Read the model definition and answer for the solid it produces. Units are mm, in the model's axes. Face numbers are marked on the shaded views. Coordinates: 2 decimals unless noted, no trailing zeros. Loops run counter-clockwise (first coordinate to the right, second up) from the corner with the lowest first, then second, coordinate; pieces in that order, holes last. Notation, with made-up numbers: (76, 62.25) -> (125, 62.25) arc R32 cw to (125, 100.25) -> close; hole circle Ø8 at (84.5, -12). An arc over 180 degrees is marked (long way). Answer in a Markdown table with one row per item.
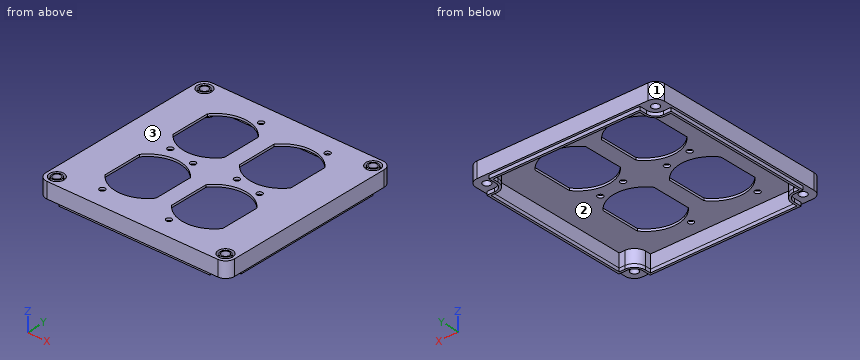
```python
from build123d import *

# Parameters (mm, degrees)
SKETCH1_W                 = 85
SKETCH1_H                 = 85
BOSS_EXTRUDE1_DEPTH       = 7
CUT_EXTRUDE4_DEPTH        = 6
FILLET4_R                 = 4
CUT_EXTRUDE1_DEPTH        = 61.510329697
SKETCH3_R                 = 1.25
CUT_EXTRUDE6_DEPTH        = 61.510329697
LPATTERN1_COUNT           = 2
LPATTERN1_PITCH           = 35
LPATTERN1_COUNT_DIR2      = 2
LPATTERN1_PITCH_DIR2      = 30
BOSS_EXTRUDE6_DEPTH       = 7
SKETCH15_R                = 1.75
CUT_EXTRUDE7_DEPTH        = 61.510329697
SKETCH30_R                = 3.25
CUT_EXTRUDE8_DEPTH        = 2
SKETCH31_R                = 2.25
SKETCH31_R_2              = 1.75
EXTRUDE_THIN2_DEPTH       = 2
MIRROR4_COPY_1_DEPTH      = 7
MIRROR4_COPY_2_SKETCH_R   = 1.75
MIRROR4_COPY_2_DEPTH      = 61.510329697
MIRROR4_COPY_3_SKETCH_R   = 3.25
MIRROR4_COPY_3_DEPTH      = 2
MIRROR4_COPY_4_SKETCH_R   = 2.25
MIRROR4_COPY_4_SKETCH_R_2 = 1.75
MIRROR4_COPY_4_DEPTH      = 2
MOVE_FACE1_BY             = 0.5
MOVE_FACE1_2_BY           = 0.5
MOVE_FACE1_3_BY           = 0.5
MOVE_FACE1_4_BY           = 0.5
MOVE_FACE1_5_BY           = 0.5
MOVE_FACE1_6_BY           = 0.5
MOVE_FACE1_7_BY           = 0.5
MOVE_FACE1_8_BY           = 0.5
MOVE_FACE1_9_BY           = 0.5
MOVE_FACE1_10_BY          = 0.5
MOVE_FACE1_11_BY          = 0.5
MOVE_FACE1_12_BY          = 0.5
EXTRUDE_THIN1_DEPTH       = 1.5


with BuildPart() as part:
    # Sketch1 → Boss-Extrude1 (new body)
    with BuildSketch(Plane.XY):
        Rectangle(SKETCH1_W, SKETCH1_H)
    extrude(amount=BOSS_EXTRUDE1_DEPTH)

    # Sketch8 → Cut-Extrude4 (cut)
    with BuildSketch(Plane(origin=(0, 0, 0), x_dir=(-1, 0, 0), z_dir=(0, 0, -1))):
        with BuildLine():
            Line((40.5, -37.5), (40.5, 37.5))
            ThreePointArc((40.5, 37.5), (39.621320344, 39.621320344), (37.5, 40.5))
            Line((37.5, 40.5), (-37.5, 40.5))
            ThreePointArc((-37.5, 40.5), (-39.621320344, 39.621320344), (-40.5, 37.5))
            Line((-40.5, 37.5), (-40.5, -37.5))
            ThreePointArc((-40.5, -37.5), (-39.621320344, -39.621320344), (-37.5, -40.5))
            Line((-37.5, -40.5), (37.5, -40.5))
            ThreePointArc((37.5, -40.5), (39.621320344, -39.621320344), (40.5, -37.5))
        make_face()
    extrude(amount=-CUT_EXTRUDE4_DEPTH, mode=Mode.SUBTRACT)

    # Fillet4
    fillet4_edges = [part.edges().sort_by_distance(p)[0] for p in [
        (42.5, -42.5, 3.5),
        (-42.5, -42.5, 3.5),
        (-42.5, 42.5, 3.5),
        (42.5, 42.5, 3.5),
    ]]
    fillet(fillet4_edges, radius=FILLET4_R)

    # Sketch2 → Cut-Extrude1 (cut, through all)
    with BuildSketch(Plane.XY.offset(7)):
        with BuildLine():
            Line((-26.5, 8.668239134), (-26.5, 26.331760866))
            ThreePointArc((-26.5, 26.331760866), (-15, 32), (-3.5, 26.331760866))
            Line((-3.5, 26.331760866), (-3.5, 8.668239134))
            ThreePointArc((-3.5, 8.668239134), (-15, 3), (-26.5, 8.668239134))
        make_face()
    cut_extrude1 = extrude(amount=-CUT_EXTRUDE1_DEPTH, mode=Mode.SUBTRACT)

    # Sketch3 → Cut-Extrude6 (cut, through all)
    with BuildSketch(Plane.XY.offset(7)):
        with Locations((-9, 34)):
            Circle(SKETCH3_R)
        with Locations((-21, 1)):
            Circle(SKETCH3_R)
    cut_extrude6 = extrude(amount=-CUT_EXTRUDE6_DEPTH, mode=Mode.SUBTRACT)

    # LPattern1: Cut-Extrude1, Cut-Extrude6 2 × 2
    with Locations(*[(j * LPATTERN1_PITCH_DIR2, -i * LPATTERN1_PITCH, 0) for i in range(LPATTERN1_COUNT) for j in range(LPATTERN1_COUNT_DIR2) if (i, j) != (0, 0)]):
        add(cut_extrude1, mode=Mode.SUBTRACT)
        add(cut_extrude6, mode=Mode.SUBTRACT)

    # Sketch14 → Boss-Extrude6 (add)
    with BuildSketch(Plane.XY.offset(7)):
        with BuildLine():
            Line((-38, 33.5), (-42.5, 33.5))
            Line((-42.5, 33.5), (-42.5, 38))
            ThreePointArc((-42.5, 38), (-41.181980515, 41.181980515), (-38, 42.5))
            Line((-38, 42.5), (-33.5, 42.5))
            Line((-33.5, 42.5), (-33.5, 38))
            ThreePointArc((-33.5, 38), (-34.818019485, 34.818019485), (-38, 33.5))
        make_face()
    boss_extrude6 = extrude(amount=-BOSS_EXTRUDE6_DEPTH)

    # Sketch15 → Cut-Extrude7 (cut, through all)
    with BuildSketch(Plane(origin=(0, 0, 0), x_dir=(-1, 0, 0), z_dir=(0, 0, -1))):
        with Locations((38, 38)):
            Circle(SKETCH15_R)
    cut_extrude7 = extrude(amount=-CUT_EXTRUDE7_DEPTH, mode=Mode.SUBTRACT)

    # Sketch30 → Cut-Extrude8 (cut)
    with BuildSketch(Plane.XY.offset(7)):
        with Locations((-38, 38)):
            Circle(SKETCH30_R)
    cut_extrude8 = extrude(amount=-CUT_EXTRUDE8_DEPTH, mode=Mode.SUBTRACT)

    # Sketch31 → Extrude-Thin2 (add)
    with BuildSketch(Plane.XY.offset(5)):
        with Locations((-38, 38)):
            Circle(SKETCH31_R)
        with Locations((-38, 38)):
            Circle(SKETCH31_R_2, mode=Mode.SUBTRACT)
    extrude_thin2 = extrude(amount=EXTRUDE_THIN2_DEPTH)

    # Mirror3: Boss-Extrude6, Cut-Extrude7, Cut-Extrude8, Extrude-Thin2 across plane
    add(boss_extrude6.mirror(Plane(origin=(0, 0, 0), x_dir=(0, 0, 1), z_dir=(1, 0, 0))))
    add(cut_extrude7.mirror(Plane(origin=(0, 0, 0), x_dir=(0, 0, 1), z_dir=(1, 0, 0))), mode=Mode.SUBTRACT)
    add(cut_extrude8.mirror(Plane(origin=(0, 0, 0), x_dir=(0, 0, 1), z_dir=(1, 0, 0))), mode=Mode.SUBTRACT)
    add(extrude_thin2.mirror(Plane(origin=(0, 0, 0), x_dir=(0, 0, 1), z_dir=(1, 0, 0))))

    # Mirror4: Boss-Extrude6, Cut-Extrude7, Cut-Extrude8, Extrude-Thin2 across plane
    add(boss_extrude6.mirror(Plane.ZX))
    add(cut_extrude7.mirror(Plane.ZX), mode=Mode.SUBTRACT)
    add(cut_extrude8.mirror(Plane.ZX), mode=Mode.SUBTRACT)
    add(extrude_thin2.mirror(Plane.ZX))

    # Mirror4 copy 1 sketch → Mirror4 copy 1 (add)
    with BuildSketch(Plane(origin=(0, 0, 7), x_dir=(-1, 0, 0), z_dir=(0, 0, 1))):
        with BuildLine():
            Line((-38, 33.5), (-42.5, 33.5))
            Line((-42.5, 33.5), (-42.5, 38))
            ThreePointArc((-42.5, 38), (-41.181980515, 41.181980515), (-38, 42.5))
            Line((-38, 42.5), (-33.5, 42.5))
            Line((-33.5, 42.5), (-33.5, 38))
            ThreePointArc((-33.5, 38), (-34.818019485, 34.818019485), (-38, 33.5))
        make_face()
    extrude(amount=-MIRROR4_COPY_1_DEPTH)

    # Mirror4 copy 2 sketch → Mirror4 copy 2 (cut, through all)
    with BuildSketch(Plane(origin=(0, 0, 0), x_dir=(1, 0, 0), z_dir=(0, 0, -1))):
        with Locations((38, 38)):
            Circle(MIRROR4_COPY_2_SKETCH_R)
    extrude(amount=-MIRROR4_COPY_2_DEPTH, mode=Mode.SUBTRACT)

    # Mirror4 copy 3 sketch → Mirror4 copy 3 (cut)
    with BuildSketch(Plane(origin=(0, 0, 7), x_dir=(-1, 0, 0), z_dir=(0, 0, 1))):
        with Locations((-38, 38)):
            Circle(MIRROR4_COPY_3_SKETCH_R)
    extrude(amount=-MIRROR4_COPY_3_DEPTH, mode=Mode.SUBTRACT)

    # Mirror4 copy 4 sketch → Mirror4 copy 4 (add)
    with BuildSketch(Plane(origin=(0, 0, 5), x_dir=(-1, 0, 0), z_dir=(0, 0, 1))):
        with Locations((-38, 38)):
            Circle(MIRROR4_COPY_4_SKETCH_R)
        with Locations((-38, 38)):
            Circle(MIRROR4_COPY_4_SKETCH_R_2, mode=Mode.SUBTRACT)
    extrude(amount=MIRROR4_COPY_4_DEPTH)

    # Move Face1: a curved face moved outward by 0.5
    add(Solid.thicken(part.faces().sort_by_distance((-34.818019485, -34.818019485, 3))[0], MOVE_FACE1_BY))

    # Move Face1 2: a face moved outward by 0.5
    extrude(part.faces().sort_by_distance((-33.5, -39.25, 3))[0], amount=MOVE_FACE1_2_BY, dir=(1, 0, 0))

    # Move Face1 3: a face moved outward by 0.5
    extrude(part.faces().sort_by_distance((-39.25, -33.5, 3))[0], amount=MOVE_FACE1_3_BY, dir=(0, 1, 0))

    # Move Face1 4: a face moved outward by 0.5
    extrude(part.faces().sort_by_distance((33.5, -39.25, 3))[0], amount=MOVE_FACE1_4_BY, dir=(-1, 0, 0))

    # Move Face1 5: a face moved outward by 0.5
    extrude(part.faces().sort_by_distance((39.25, -33.5, 3))[0], amount=MOVE_FACE1_5_BY, dir=(0, 1, 0))

    # Move Face1 6: a curved face moved outward by 0.5
    add(Solid.thicken(part.faces().sort_by_distance((34.818019485, -34.818019485, 3))[0], MOVE_FACE1_6_BY))

    # Move Face1 7: a face moved outward by 0.5
    extrude(part.faces().sort_by_distance((33.5, 39.25, 3))[0], amount=MOVE_FACE1_7_BY, dir=(-1, 0, 0))

    # Move Face1 8: a curved face moved outward by 0.5
    add(Solid.thicken(part.faces().sort_by_distance((34.818019485, 34.818019485, 3))[0], MOVE_FACE1_8_BY))

    # Move Face1 9: a face moved outward by 0.5
    extrude(part.faces().sort_by_distance((39.25, 33.5, 3))[0], amount=MOVE_FACE1_9_BY, dir=(0, -1, 0))

    # Move Face1 10: a face moved outward by 0.5
    extrude(part.faces().sort_by_distance((-39.25, 33.5, 3))[0], amount=MOVE_FACE1_10_BY, dir=(0, -1, 0))

    # Move Face1 11: a curved face moved outward by 0.5
    add(Solid.thicken(part.faces().sort_by_distance((-34.818019485, 34.818019485, 3))[0], MOVE_FACE1_11_BY))

    # Move Face1 12: a face moved outward by 0.5
    extrude(part.faces().sort_by_distance((-33.5, 39.25, 3))[0], amount=MOVE_FACE1_12_BY, dir=(1, 0, 0))

    # Sketch29 → Extrude-Thin1 (add)
    with BuildSketch(Plane(origin=(0, 0, 0), x_dir=(-1, 0, 0), z_dir=(0, 0, -1))):
        with BuildLine():
            Line((34, 38), (34, 41.5))
            Line((34, 41.5), (-34, 41.5))
            Line((-34, 41.5), (-34, 38))
            ThreePointArc((-34, 38), (-35.171572875, 35.171572875), (-38, 34))
            Line((-38, 34), (-41.5, 34))
            Line((-41.5, 34), (-41.5, -34))
            Line((-41.5, -34), (-38, -34))
            ThreePointArc((-38, -34), (-35.171572875, -35.171572875), (-34, -38))
            Line((-34, -38), (-34, -41.5))
            Line((-34, -41.5), (34, -41.5))
            Line((34, -41.5), (34, -38))
            ThreePointArc((34, -38), (35.171572875, -35.171572875), (38, -34))
            Line((38, -34), (41.5, -34))
            Line((41.5, -34), (41.5, 34))
            Line((41.5, 34), (38, 34))
            ThreePointArc((38, 34), (35.171572875, 35.171572875), (34, 38))
        make_face()
        with BuildLine():
            Line((33, 38), (33, 40.5))
            Line((33, 40.5), (-33, 40.5))
            Line((-33, 40.5), (-33, 38))
            ThreePointArc((-33, 38), (-34.464466094, 34.464466094), (-38, 33))
            Line((-38, 33), (-40.5, 33))
            Line((-40.5, 33), (-40.5, -33))
            Line((-40.5, -33), (-38, -33))
            ThreePointArc((-38, -33), (-34.464466094, -34.464466094), (-33, -38))
            Line((-33, -38), (-33, -40.5))
            Line((-33, -40.5), (33, -40.5))
            Line((33, -40.5), (33, -38))
            ThreePointArc((33, -38), (34.464466094, -34.464466094), (38, -33))
            Line((38, -33), (40.5, -33))
            Line((40.5, -33), (40.5, 33))
            Line((40.5, 33), (38, 33))
            ThreePointArc((38, 33), (34.464466094, 34.464466094), (33, 38))
        make_face(mode=Mode.SUBTRACT)
    extrude(amount=EXTRUDE_THIN1_DEPTH)


solid = part.part
```
1. A cutting plane is placed at C-C on x = 17. Give the vertices of the cut face in (y, z), and give its area (3 significant figures).
A:
| item | result |
|---|---|
| outline | (-42.5, 0) -> (-41.5, 0) -> (-41.5, -1.5) -> (-40.5, -1.5) -> (-40.5, 6) -> (-31.86, 6) -> (-31.86, 7) -> (-42.5, 7) -> close; (-3.14, 6) -> (3.14, 6) -> (3.14, 7) -> (-3.14, 7) -> close; (31.86, 6) -> (40.5, 6) -> (40.5, -1.5) -> (41.5, -1.5) -> (41.5, 0) -> (42.5, 0) -> (42.5, 7) -> (31.86, 7) -> close |
| area | 54.6 mm2 |
2. Find the intervals of material crossed by probe 1 along X at (y, z) = (-19.5, 6.25); probe 2 along X at (y, z) = (38, 1.5); probe 3 along X at (y, z) = (-15, 5.75), in increasing order.
A:
| item | result |
|---|---|
| probe 1 | x = -42.5 to -26.5, -3.5 to 3.5, 26.5 to 42.5 |
| probe 2 | x = -42.5 to -39.75, -36.25 to -33, 33 to 36.25, 39.75 to 42.5 |
| probe 3 | x = -42.5 to -40.5, 40.5 to 42.5 |
3. A cutting plane is placed at B-B on z = 2.75. Give the vertices of the cut face in (x, y), and give its area (3 significant figures).
A:
| item | result |
|---|---|
| outline | (-42.5, -38.5) arc R4 ccw to (-38.5, -42.5) -> (38.5, -42.5) arc R4 ccw to (42.5, -38.5) -> (42.5, 38.5) arc R4 ccw to (38.5, 42.5) -> (-38.5, 42.5) arc R4 ccw to (-42.5, 38.5) -> close; hole (-40.5, -33) -> (-38, -33) arc R5 cw to (-33, -38) -> (-33, -40.5) -> (33, -40.5) -> (33, -38) arc R5 cw to (38, -33) -> (40.5, -33) -> (40.5, 33) -> (38, 33) arc R5 cw to (33, 38) -> (33, 40.5) -> (-33, 40.5) -> (-33, 38) arc R5 cw to (-38, 33) -> (-40.5, 33) -> close; hole circle Ø3.5 at (-38, -38); hole circle Ø3.5 at (-38, 38); hole circle Ø3.5 at (38, -38); hole circle Ø3.5 at (38, 38) |
| area | 815 mm2 |
4. A cutting plane is placed at A-A on y = 17. Give the vertices of the cut face in (x, z).
A:
| item | result |
|---|---|
| outline | (-42.5, 0) -> (-41.5, 0) -> (-41.5, -1.5) -> (-40.5, -1.5) -> (-40.5, 6) -> (-26.5, 6) -> (-26.5, 7) -> (-42.5, 7) -> close; (-3.5, 6) -> (3.5, 6) -> (3.5, 7) -> (-3.5, 7) -> close; (26.5, 6) -> (40.5, 6) -> (40.5, -1.5) -> (41.5, -1.5) -> (41.5, 0) -> (42.5, 0) -> (42.5, 7) -> (26.5, 7) -> close |
5. A cutting plane is placed at D-D on x = 27.5. Give the vertices of the cut face in (y, z), and give its area (3 significant figures).
A:
| item | result |
|---|---|
| outline | (-42.5, 0) -> (-41.5, 0) -> (-41.5, -1.5) -> (-40.5, -1.5) -> (-40.5, 6) -> (40.5, 6) -> (40.5, -1.5) -> (41.5, -1.5) -> (41.5, 0) -> (42.5, 0) -> (42.5, 7) -> (-42.5, 7) -> close |
| area | 112 mm2 |
6. Given pin 1 Ø1.6 at (y, z) = (39.5, -0.5) entering from -X; pin 2 Ø3 at (x, y) = (-21, 1) entering from -Z; pin 3 Ø4 at (x, y) = (-38, -38) entering from -Z, each flat-ended and moving along its own axis, determine where each tip first touches the part or whether it passes through.
A:
| item | result |
|---|---|
| pin 1 | stops at x = -42.48 |
| pin 2 | stops at z = 6 |
| pin 3 | stops at z = 0 |
7. The mould has two halves that part along Y. Classify the marked faces 1, 2 and 3: pulls with the +Y half, pulls with the -Y half, needs draft (parallel to the pull), parting line crosses it, or undercut.
A:
| item | result |
|---|---|
| face 1 | pulls with the +Y half |
| face 2 | undercut |
| face 3 | needs draft |
